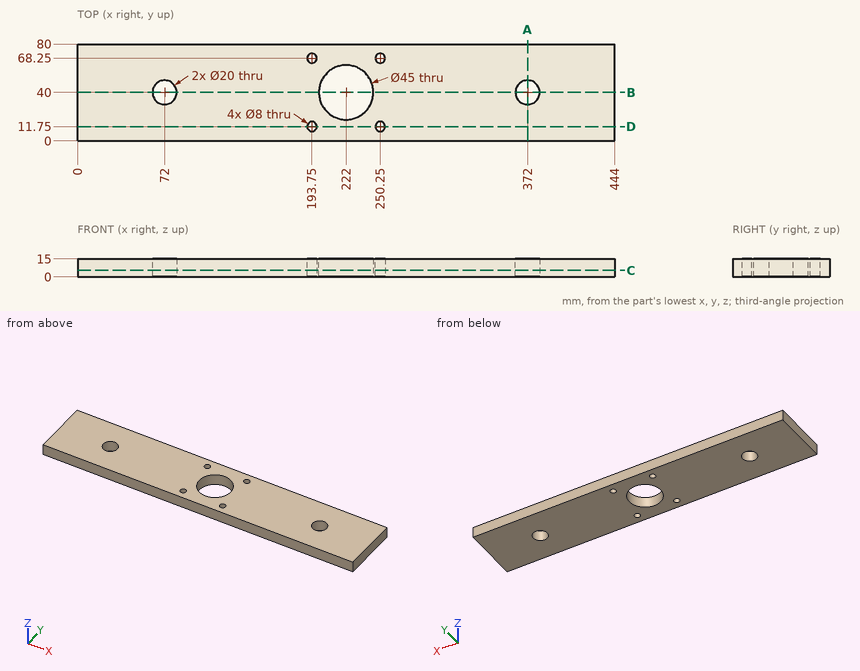
Here's the drawing with two shaded views (mm, measured from the low corner). I have some questions. Give positions to 0.01 mm unless a question says otherwise; leave off trailing zeros. Write each loop counter-clockwise with the first axis right and the second up, starting at its lowest first coordinate (ties: lowest second). Pieces come first, ordered by that corner, then holes. Notation, with made-up numbers: (-34.75, 30.25) - (-10.75, 30.25) arc R20 cw to (-10.75, 49.25) - close; hole circle Ø5 at (6.25, 16). An arc over 180 degrees is marked (long way). One line per item, written item: value. Start each with the question number.
Item 1: Please list where these lines run through material, in increasing order: line 1 (Y direction, x = 72, z = 9); line 2 (Y direction, x = 250.25, z = 5.75); line 3 (X direction, y = 36, z = 6.5). Write a range as from..to.
Item 2: Imagine slicing it at A-A, the plane x = 372. List the corners of the cut face in (y, z) for me, and give its area (3 significant figures).
Item 3: Imagine slicing it at C-C, the plane z = 5.5. List the corners of the cut face in (x, y) for me, and give its area (3 significant figures).
Item 4: I'm going to push a flat-ended pin straight in: pin 1 (7 mm diameter, centred on x = 250.25, y = 11.75, fed in from +Z). Where does the tip first touch, or does it pass through?
Item 5: Imagine slicing it at B-B, the plane y = 40. List the corners of the cut face in (x, z) for me, and give its area (4 significant figures).
Item 6: Imagine slicing it at D-D, the plane y = 11.75. List the corners of the cut face in (x, z) for me.
Geometry says:
1. line 1: 0..30, 50..80
1. line 2: 0..7.75, 15.75..64.25, 72.25..80
1. line 3: 0..62.83, 81.17..199.86, 244.14..362.83, 381.17..444
2. outline: (0, 0) - (30, 0) - (30, 15) - (0, 15) - close; (50, 0) - (80, 0) - (80, 15) - (50, 15) - close
2. area: 900 mm^2
3. outline: (0, 0) - (444, 0) - (444, 80) - (0, 80) - close; hole circle Ø20 at (72, 40); hole circle Ø8 at (193.75, 11.75); hole circle Ø8 at (193.75, 68.25); hole circle Ø45 at (222, 40); hole circle Ø8 at (250.25, 11.75); hole circle Ø8 at (250.25, 68.25); hole circle Ø20 at (372, 40)
3. area: 33,100 mm^2
4. pin 1: through
5. outline: (0, 0) - (62, 0) - (62, 15) - (0, 15) - close; (82, 0) - (199.5, 0) - (199.5, 15) - (82, 15) - close; (244.5, 0) - (362, 0) - (362, 15) - (244.5, 15) - close; (382, 0) - (444, 0) - (444, 15) - (382, 15) - close
5. area: 5,385 mm^2
6. outline: (0, 0) - (189.75, 0) - (189.75, 15) - (0, 15) - close; (197.75, 0) - (246.25, 0) - (246.25, 15) - (197.75, 15) - close; (254.25, 0) - (444, 0) - (444, 15) - (254.25, 15) - close
